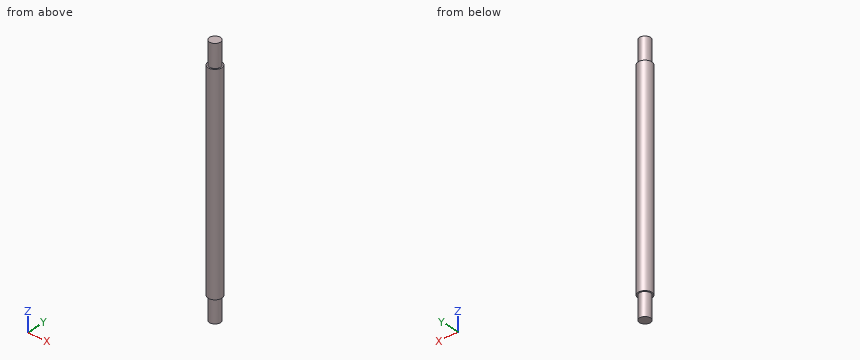
Autodesk Inventor part; units mm, degrees
ref_plane "YZ Plane" through (0, 0, 0) normal (1, 0, 0) x (0, 1, 0)
ref_plane "XZ Plane" through (0, 0, 0) normal (0, 1, 0) x (-1, 0, 0)
ref_plane "XY Plane" through (0, 0, 0) normal (0, 0, 1) x (1, 0, 0)
sketch "Sketch1" plane through (0, 0, 0) normal (0, 0, 1) x (1, 0, 0)
  circle A0 centre (0, 0) radius 10
  dimension "d0" = 20
extrude "Extrusion1" add sketch "Sketch1" along normal blind 151.65
sketch "Sketch2" plane through (0, 0, 0) normal (0, 0, -1) x (-1, 0, 0)
  circle A0 centre (0, 0) radius 8
  dimension "d3" = 16
extrude "Extrusion2" add sketch "Sketch2" along normal blind 33
mirror "Mirror1" about plane through (0, 0, 151.65) normal (0, 0, 1) of "Extrusion1", "Extrusion2"
properties part number "BielaConexion"
CAD build for the part. Positions are in the model's coordinates, mm. Coordinates: 2 decimals unless noted, no trailing zeros. Order: outer loops, then holes, each group sorted by start corner. A loop starts at its lowest first (then second) coordinate and runs counter-clockwise, first axis right, second up. Notation, with made-up numbers: (4, 0.25) - (62, 0.25) arc R37 cw to (62, 37.25) - close; hole circle Ø1 at (-8.75, 9). An arc over 180 degrees is marked (long way). Use a Markdown table: item, result. Add a question column.
(1) Saw through at B-B (y = 4.25). Give the cut face in (x, z).
(2) Drill centre lines: line 1 along Y through (x, z) = (1, -9.5); line 2 along Y through (x, z) = (-1, 216); line 3 along X through (y, z) = (-6, 196). Where is each one in solid material? Low to high. Write a range as [from, to].
(3) Saw through at A-A (x = 0). Give the cut face in (y, z), then the cut area to 3 significant figures.
(4) Saw through at C-C (z = 24.5). Give the cut face in (x, y), then the cut area to 3 significant figures.
(5) Flat gauge pins, fed straight in: pin 1 (3 mm diameter, centred on x = 3.5, z = 157.5, fed in from -Y); pin 2 (1.5 mm diameter, centred on y = 4.5, z = 225.5, fed in from -X); pin 3 (5 mm diameter, centred on y = 2, z = 70, fed in from +X); pin 4 (1 mm diameter, centred on y = 7, z = 281, fed in from +X). Where does each tip first touch, or does it go through?
Solved:
| question | item | result |
|---|---|---|
| 1 | outline | (-9.05, 0) - (-6.78, 0) - (-6.78, -33) - (6.78, -33) - (6.78, 0) - (9.05, 0) - (9.05, 303.3) - (6.78, 303.3) - (6.78, 336.3) - (-6.78, 336.3) - (-6.78, 303.3) - (-9.05, 303.3) - close |
| 2 | line 1 | y = [-7.94, 7.94] |
| 2 | line 2 | y = [-9.95, 9.95] |
| 2 | line 3 | x = [-8, 8] |
| 3 | outline | (-10, 0) - (-8, 0) - (-8, -33) - (8, -33) - (8, 0) - (10, 0) - (10, 303.3) - (8, 303.3) - (8, 336.3) - (-8, 336.3) - (-8, 303.3) - (-10, 303.3) - close |
| 3 | area | 7,120 mm² |
| 4 | outline | circle Ø20 at (0, 0) |
| 4 | area | 314 mm² |
| 5 | pin 1 | stops at y = -9.8 |
| 5 | pin 2 | stops at x = -9.27 |
| 5 | pin 3 | stops at x = 10 |
| 5 | pin 4 | stops at x = 7.6 |
